Can you work these out from the model? Positions are in its coordinate system, mm. A direction names the side the tool comes from. Give positions to 0.01 mm unless a question says otherwise; leave off trailing zeros. Write each loop counter-clockwise with the first axis right and the second up, starting at its lowest first coordinate (ties: lowest second). Pieces come first, ordered by that corner, then holes.
from build123d import *
from build123d.topology import SkipClean

# Parameters (mm, degrees)
SWEEP1_PITCH       = 5
SWEEP1_HEIGHT      = 2.25
SWEEP1_RADIUS      = 3.15
SWEEP1_START_ANGLE = 180
SKETCH3_W          = 0.65
SKETCH3_H          = 1
SKETCH4_W          = 0.868914335
SKETCH4_H          = 0.369387361
SKETCH4_W_2        = 0.738311658
SKETCH4_H_2        = 0.690928268


with BuildPart() as part:
    # Sketch1 → Revolve1 (revolve)
    with BuildSketch(Plane(origin=(0, 0, 0), x_dir=(1, 0, 0), z_dir=(0, 1, 0)), mode=Mode.PRIVATE) as revolve1_sk:
        Polygon((-0.24, 0), (-0.725, 0), (-2.175, 17.35), (-2.25, 17.35), (-2.65, 28.75), (-3.15, 28.75), (-3.15, 32.35), (-2.1, 32.35), (-2.1, 28.75), (-1.655636817, 17.738125355), (-0.862390363, 17.738125355), align=None)
    revolve(revolve1_sk.sketch.rotate(Axis((0, 0, 1.904272973), (0, 0, -1)), 180), axis=Axis((0, 0, 1.904272973), (0, 0, -1)))

    # Sweep1: sweep along a helix
    with BuildLine() as sweep1_path:
        add(Helix(SWEEP1_PITCH, SWEEP1_HEIGHT, SWEEP1_RADIUS, center=(0, 0, -32.35), direction=(0, 0, 1), mode=Mode.PRIVATE).rotate(Axis((0, 0, -32.35), (0, 0, 1)), SWEEP1_START_ANGLE))
    # Sketch3 → Sweep1 (sweep)
    with BuildSketch(Plane(origin=(0, 0, 0), x_dir=(1, 0, 0), z_dir=(0, 1, 0))):
        with Locations((-3.475, 31.85)):
            Rectangle(SKETCH3_W, SKETCH3_H)
        with Locations((3.475, 31.85)):
            Rectangle(SKETCH3_W, SKETCH3_H)
    sweep(path=sweep1_path.line, is_frenet=True)

    # Sketch4 → Cut-Revolve1 (revolve, cut)
    with SkipClean():  # the faces are left unmerged after this step: merging them gives an invalid solid
        with BuildSketch(Plane(origin=(0, 0, 0), x_dir=(1, 0, 0), z_dir=(0, 1, 0))):
            with Locations((-3.584457168, 32.16530632)):
                Rectangle(SKETCH4_W, SKETCH4_H)
            with Locations((-3.519155829, 29.095464134)):
                Rectangle(SKETCH4_W_2, SKETCH4_H_2)
        revolve(axis=Axis((0, 0, -32.799017305), (0, 0, 1)), mode=Mode.SUBTRACT)


solid = part.part
(1) Will these pins go through, and if not, where does the flat tip stop? P1, Ø0.5, axis at x = 3.5, z = -31.5, coming from the -Y side; P2, Ø1.5, axis at y = 0, z = -5.5, coming from the +X side; P3, Ø1, axis at x = 0, y = 0.5, coming from the -Z side.
Returned:
P1: stops at y = 0
P2: stops at x = 1.25
P3: stops at z = -17.74
(2) For faces 1 (the face through (2.003, -0.631, -30.525)), 2 (the face through (3, -2, -29.441)), 3 (the face through (-3, 2, -29.441)), 4 (the face through (-3.4, -0.9, -31.981)), 5 (the face through (3.3, 0.8, -31.981)), which set-ups out of +Z, -Z, +X, -X, +Y, -Y let a thin tool reach every point of the face, with its end or its side?
Returned:
face 1: -Z
face 2: +Z, +X, -Y
face 3: +Z, -X, +Y
face 4: -Z, -X, -Y
face 5: -Z, +X, +Y
(3) If we mould it in two halves opening along X, with no side actions, what happens to faces 6 (the face through (-0.119, 0.534, -8.745)), 7 (the face through (-0.19, -1.45, -8.8)), 8 (the face through (2, -2, -28.75))? For each: +X half, -X half, draft (parallel to the pull), parting line (faces both ways), or undercut.
Returned:
face 6: undercut
face 7: parting line
face 8: draft
(4) If I drill on L1, parallel to Y at x = 0, z = -31.6; L2, parallel to Y at x = 0, z = -30.8; L3, parallel to Z at x = -0.75, y = 2.75, over which ranges is the centre line in solid material (lowest first)?
Returned:
L1: y = -3.15 to -2.1, 2.1 to 3.15
L2: y = -3.8 to -2.1, 2.1 to 3.8
L3: z = -32.35 to -28.75
(5) Imagine slicing it at B-B, the plane z = -7.5. Write out the boundary of the cut face in (x, y).
Returned:
outline: circle Ø2.7 at (0, 0); hole circle Ø1.01 at (0, 0)
(6) Imagine slicing it at A-A, the plane z = -14. Write out the boundary of the cut face in (x, y).
Returned:
outline: circle Ø3.79 at (0, 0); hole circle Ø1.46 at (0, 0)
